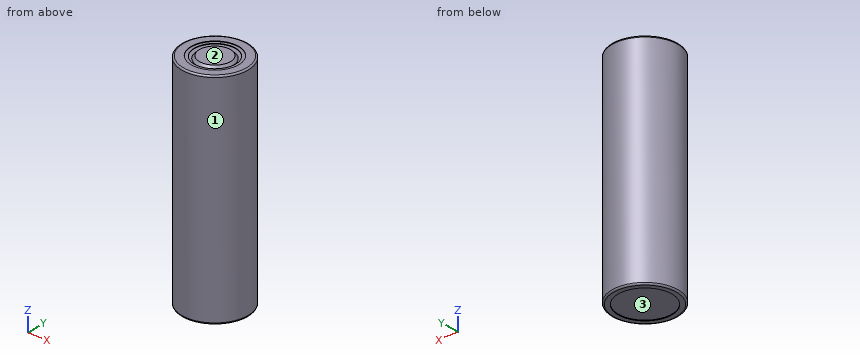
from build123d import *

# Parameters (mm, degrees)
SKETCH1_R           = 10.65
BOSS_EXTRUDE1_DEPTH = 70.4
SKETCH2_R           = 8.65
CUT_EXTRUDE1_DEPTH  = 0.2
FILLET1_R           = 0.5


with BuildPart() as part:
    # Sketch1 → Boss-Extrude1 (new body)
    with BuildSketch(Plane.XY):
        Circle(SKETCH1_R)
    extrude(amount=BOSS_EXTRUDE1_DEPTH)

    # Sketch2 → Cut-Extrude1 (cut)
    with BuildSketch(Plane.XY):
        Circle(SKETCH2_R)
    extrude(amount=CUT_EXTRUDE1_DEPTH, mode=Mode.SUBTRACT)

    # Sketch3 → Cut-Revolve1 (revolve, cut)
    with BuildSketch(Plane(origin=(0, 0, 0), x_dir=(1, 0, 0), z_dir=(0, 1, 0))):
        Polygon((-9.149999999, -70.1), (-9.149999999, -69.600000001), (-5.799999999, -69.600000001), (-5, -70.4), (-7.650000002, -70.4), (-7.650000002, -70.25), (-6.649999999, -70.25), (-6.649999999, -70.1), align=None)
    revolve(axis=Axis((0, 0, 70.4), (0, 0, -1)), mode=Mode.SUBTRACT)

    # Fillet1
    fillet1_edges = [part.edges().sort_by_distance(p)[0] for p in [
        (-10.65, 0, 0),
        (-10.65, 0, 70.4),
    ]]
    fillet(fillet1_edges, radius=FILLET1_R)


solid = part.part
Input: part model. Units: mm. Frame: model coordinates. Face numbers are marked on the shaded views. Coordinates: 2 decimals unless noted, no trailing zeros. Order: outer loops, then holes, each group sorted by start corner. A loop starts at its lowest first (then second) coordinate and runs counter-clockwise, first axis right, second up. Notation, with made-up numbers: M 29,66.25 L 68,66.25 A12 ccw 68,88.25 Z; hole C 9.5,-40 d7. An arc over 180 degrees is marked long. Write item = value, one per line. Start each with the question number.
(1) First-contact query: P1, Ø5, axis at x = 0.5, y = 0.5, coming from the -Z side; P2, Ø1.5, axis at y = -1.5, z = 42, coming from the -X side; P3, Ø2, axis at x = 4, z = 12.5, coming from the -Y side. Flat tips, straight axial feed; report the tip coordinate or a pass-through.
(2) Section A-A on z = 8.5. Output: boundary loops of the cut face in (x, y).
(3) Pull-direction query (Y, two-part tool) for the marked faces 1, 2 and 3; classes: released by +Y, released by -Y, zero draft, split by the parting line, or undercut.
(4) Line query: line 1 along Z through (x, y) = (7, 5.75); line 2 along Y through (x, z) = (0, 69.7); line 3 along Z through (x, y) = (3.5, -7.5). Output: solid intervals per line, ascending. Write a range as [from, to].
Result set:
q1.P1 = 0.2
q1.P2 = -10.62
q1.P3 = -10.22
q2.outline = C 0,0 d21.3
q3.face_1 = split by the parting line
q3.face_2 = zero draft
q3.face_3 = undercut
q4.line_1 = [0, 69.6], [70.1, 70.4]
q4.line_2 = [-10.65, -9.15], [-5.7, 5.7], [9.15, 10.65]
q4.line_3 = [0.2, 69.6], [70.1, 70.4]
